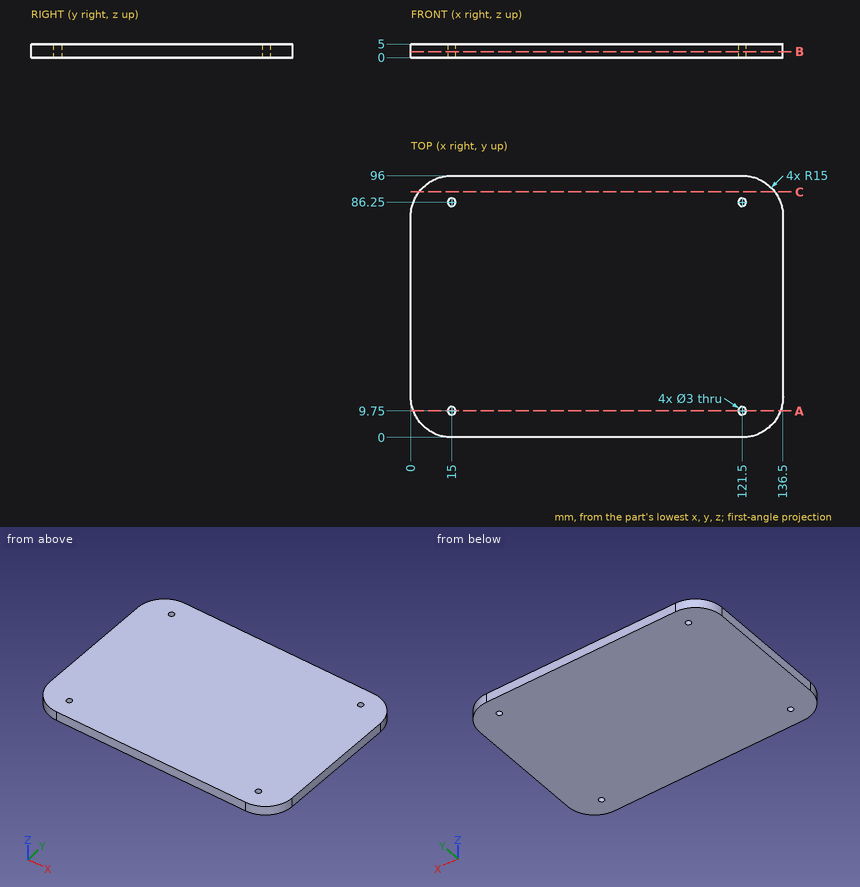
Study the drawing (mm; zero at the part's minimum x, y, z) and answer. Give positions to 0.01 mm unless a question says otherwise; leave off trailing zeros. Loops run counter-clockwise (first coordinate to the right, second up) from the corner with the lowest first, then second, coordinate; pieces in that order, holes last. Notation, with made-up numbers: (69, 30) - (126, 30) arc R17 cw to (126, 34) - close; hole circle Ø10 at (-25, 70.25). An arc over 180 degrees is marked (long way). Return JSON: item names as keys, results as strings. Group by question number.
1. Find section A-A (y = 9.75). Write down the section's boundary in (x, z), then the cut area to 3 significant figures.
2. Find section C-C (y = 90). Write down the section's boundary in (x, z).
3. Given pin 1 Ø1 at (y, z) = (13.5, 0.5) entering from -X, flat-ended and moving along its own axis, determine where the tip first touches the part or whether it passes through.
4. Straight lines are drawn through the part: line 1 (X direction, y = 86.25, z = 1.3); line 2 (X direction, y = 10.5, z = 2.55); line 3 (Y direction, x = 16, z = 4.7). For each, find the intervals that lie inside material, in ascending order. Write a range as [from, to].
5. Find section B-B (z = 2.2). Write down the section's boundary in (x, y), then the cut area to 3 significant figures.
Verdict:
{
 "1": {"outline": "(0.95, 0) - (13.5, 0) - (13.5, 5) - (0.95, 5) - close; (16.5, 0) - (120, 0) - (120, 5) - (16.5, 5) - close; (123, 0) - (135.55, 0) - (135.55, 5) - (123, 5) - close", "area": "643 mm^2"},
 "2": {"outline": "(3, 0) - (133.5, 0) - (133.5, 5) - (3, 5) - close"},
 "3": {"pin 1": "stops at x = 0.03"},
 "4": {"line 1": "x = [0.95, 13.5], [16.5, 120], [123, 135.55]", "line 2": "x = [0.69, 13.7], [16.3, 120.2], [122.8, 135.81]", "line 3": "y = [0, 8.63], [10.87, 85.13], [87.37, 96]"},
 "5": {"outline": "(0, 15) arc R15 ccw to (15, 0) - (121.5, 0) arc R15 ccw to (136.5, 15) - (136.5, 81) arc R15 ccw to (121.5, 96) - (15, 96) arc R15 ccw to (0, 81) - close; hole circle Ø3 at (15, 9.75); hole circle Ø3 at (15, 86.25); hole circle Ø3 at (121.5, 9.75); hole circle Ø3 at (121.5, 86.25)", "area": "12,900 mm^2"}
}
